Work out the finished part from the listing and answer in its coordinate system (mm). A direction names the side the tool comes from. Give positions to 0.01 mm unless a question says otherwise; leave off trailing zeros. Loops run counter-clockwise (first coordinate to the right, second up) from the corner with the lowest first, then second, coordinate; pieces in that order, holes last. Notation, with made-up numbers: M 46,35 L 79,35 A16 cw 79,59 Z; hole C -5,81.5 d4. An arc over 180 degrees is marked long. Use a Markdown table: item, result.
```python
from build123d import *

# Parameters (mm, degrees)
SKETCH1_W           = 30.5
SKETCH1_H           = 8
SKETCH1_R           = 2.1
BOSS_EXTRUDE1_DEPTH = 21
CUT_EXTRUDE1_DEPTH  = 17.5
SKETCH4_R           = 2.1
CUT_EXTRUDE3_DEPTH  = 38.5
SKETCH6_R           = 2.1
BOSS_EXTRUDE3_DEPTH = 2
SKETCH7_R           = 2.1
BOSS_EXTRUDE4_DEPTH = 3


with BuildPart() as part:
    # Sketch1 → Boss-Extrude1 (new body)
    with BuildSketch(Plane(origin=(0, 0, 0), x_dir=(1, 0, 0), z_dir=(0, 1, 0))):
        with Locations((3.75, 0)):
            Rectangle(SKETCH1_W, SKETCH1_H)
        with Locations(Location((0, 0, 0), (0, 0, 90))):
            Circle(SKETCH1_R, mode=Mode.SUBTRACT)
        with Locations(Location((-7.5, 0, 0), (0, 0, 90))):
            Circle(SKETCH1_R, mode=Mode.SUBTRACT)
        with Locations(Location((7.5, 0, 0), (0, 0, 90))):
            Circle(SKETCH1_R, mode=Mode.SUBTRACT)
        with Locations(Location((15, 0, 0), (0, 0, 90))):
            Circle(SKETCH1_R, mode=Mode.SUBTRACT)
    extrude(amount=BOSS_EXTRUDE1_DEPTH)

    # Sketch2 → Cut-Extrude1 (cut)
    with BuildSketch(Plane.XY.offset(4)):
        Polygon((12.8, 21), (1.738392209, 10), (-9.200343126, 21), align=None)
    extrude(amount=-CUT_EXTRUDE1_DEPTH, mode=Mode.SUBTRACT)

    # Sketch4 → Cut-Extrude3 (cut)
    with BuildSketch(Plane(origin=(19, 0, 0), x_dir=(0, 0, -1), z_dir=(1, 0, 0))):
        with Locations((0, 4)):
            Circle(SKETCH4_R)
    extrude(amount=-CUT_EXTRUDE3_DEPTH, mode=Mode.SUBTRACT)

    # Sketch6 → Boss-Extrude3 (add)
    with BuildSketch(Plane.XZ):
        with Locations(Location((-7.5, 0, 0), (0, 0, 270))):
            Circle(SKETCH6_R)
        with Locations(Location((0, 0, 0), (0, 0, 270))):
            Circle(SKETCH6_R)
        with Locations(Location((7.5, 0, 0), (0, 0, 270))):
            Circle(SKETCH6_R)
        with Locations(Location((15, 0, 0), (0, 0, 90))):
            Circle(SKETCH6_R)
    extrude(amount=-BOSS_EXTRUDE3_DEPTH)

    # Sketch7 → Boss-Extrude4 (add)
    with BuildSketch(Plane(origin=(19, 0, 0), x_dir=(0, 0, -1), z_dir=(1, 0, 0))):
        with Locations((0, 4)):
            Circle(SKETCH7_R)
    extrude(amount=-BOSS_EXTRUDE4_DEPTH)


solid = part.part
```
(1) A cutting plane is placed at C-C (x = 14). Write down the section's boundary in (y, z).
Entries:
| item | result |
|---|---|
| outline | M 0,-4 L 21,-4 L 21,-1.85 L 5,-1.85 A2.1 cw 3,-1.85 L 2,-1.85 L 2,1.85 L 3,1.85 A2.1 cw 5,1.85 L 21,1.85 L 21,4 L 0,4 Z |
(2) A cutting plane is placed at B-B (z = 3). Write down the section's boundary in (x, y), and give its area (3 significant figures).
Entries:
| item | result |
|---|---|
| outline | M -11.5,0 L 19,0 L 19,21 L 12.8,21 L 1.74,10 L -9.2,21 L -11.5,21 Z |
| area | 519 mm² |
(3) The mould has two halves that part along Y. Classify faces 1 (the cylindrical face through (16.4, 2.27, -1.19)), 2 (the flat face through (-7, 2, 0)), 3 (the cylindrical face through (-9.582, 12.381, 0.273)), 4 (the flat face through (4, 0, 0)): released by +Y, released by -Y, zero draft, split by the parting line, or undercut.
Entries:
| item | result |
|---|---|
| face 1 | undercut |
| face 2 | released by +Y |
| face 3 | zero draft |
| face 4 | released by -Y |
(4) A cutting plane is placed at D-D (x = 4). Write down the section's boundary in (y, z), and give its area (3 significant figures).
Entries:
| item | result |
|---|---|
| outline | M 0,-4 L 12.25,-4 L 12.25,4 L 0,4 Z; hole C 4,0 d4.2 |
| area | 84.1 mm² |
(5) Which of the six approach directions +Z, -Z, +X, -X, +Y, -Y give full straight-line access (tool end or side, diameter ignored) to faces 5 (the flat face through (-10, 21, 0)), 6 (the cylindrical face through (9.55, 10.84, 0.46)), 7 (the flat face through (6.118, 14.355, 1.834))?
Entries:
| item | result |
|---|---|
| face 5 | +Z, -Z, +X, -X, +Y |
| face 6 | +Y |
| face 7 | +Z, -Z, +Y |
(6) Given P1, Ø4, axis at x = 7.5, z = 0, coming from the +Y side; P2, Ø2.5, axis at x = 15, z = 0, coming from the +Y side; P3, Ø1.2, axis at y = 3.5, z = 1, coming from the -X side, each flat-ended and moving along its own axis, determine where each tip first touches the part or whether it passes through.
Entries:
| item | result |
|---|---|
| P1 | stops at y = 2 |
| P2 | stops at y = 6.1 |
| P3 | stops at x = 16 |
(7) A cutting plane is placed at A-A (y = 19.75). Write down the section's boundary in (x, z).
Entries:
| item | result |
|---|---|
| outline | M -11.5,-4 L -7.96,-4 L -7.96,-2.05 A2.1 cw -7.96,2.05 L -7.96,4 L -11.5,4 Z; M 11.54,-4 L 19,-4 L 19,4 L 11.54,4 Z; hole C 15,0 d4.2 |
(8) Consider probe 1 along X at (y, z) = (8.75, 0); probe 2 along Z at (x, y) = (7.5, 14); probe 3 along X at (y, z) = (12.75, 0). Determine where each line is inside the solid, lowest interval first. Write a range as [from, to].
Entries:
| item | result |
|---|---|
| probe 1 | x = [-11.5, -9.6], [-5.4, -2.1], [2.1, 5.4], [9.6, 12.9], [17.1, 19] |
| probe 2 | z = [-4, -2.1], [2.1, 4] |
| probe 3 | x = [-11.5, -9.6], [-5.4, -2.1], [4.5, 5.4], [9.6, 12.9], [17.1, 19] |
